For this review, use the dimensioned drawing (mm, ordinates from the lowest corner) and the shaded views. A direction names the side the tool comes from. Coordinates: 2 decimals unless noted, no trailing zeros. Loops run counter-clockwise (first coordinate to the right, second up) from the corner with the lowest first, then second, coordinate; pieces in that order, holes last.
1. Take a section at D-D, the plane x = 37. State the section outline as (y, z) points, then the cut area to 3 significant figures.
2. Take a section at B-B, the plane y = 2.3. State the section outline as (x, z) points.
3. Clearance check with flat-ended pins moving along their axes: P1, Ø1, axis at y = 2, z = 6, coming from the +X side; P2, Ø1, axis at y = 3.5, z = 13.5, coming from the +X side; P3, Ø3, axis at y = 0.5, z = 15.5, coming from the +X side. State where each tip first meets the part, or that it passes through.
4. Take a section at C-C, the plane z = 8.5. State the section outline as (x, y) points.
5. To check wall thickness, follow probe 1 along X at (y, z) = (1.05, 2); probe 2 along X at (y, z) = (3.15, 8.25); probe 3 along Z at (x, y) = (43, 1.9). State the ranges of each line that lie inside material, in increasing order.
6. Take a section at A-A, the plane z = 3.5. State the section outline as (x, y) points.
7. Machinability: for the marked faces 1, 2, 3, 4 and 5, which of the approach directions +Z, -Z, +X, -X, +Y, -Y give a long, thin tool a straight path to every point of the face, cutting with its end or side? Answer none if there is none.
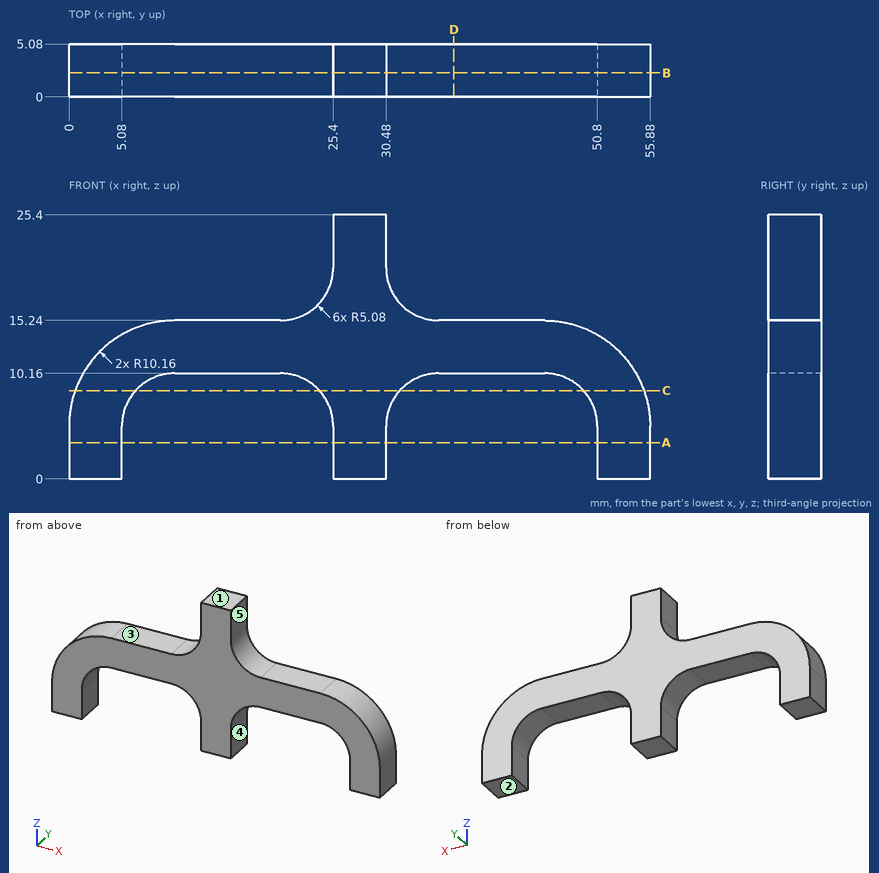
Results list:
1. outline: (0, 10.16) - (5.08, 10.16) - (5.08, 15.24) - (0, 15.24) - close
1. area: 25.8 mm2
2. outline: (0, 0) - (5.08, 0) - (5.08, 5.08) arc R5.08 cw to (10.16, 10.16) - (20.32, 10.16) arc R5.08 cw to (25.4, 5.08) - (25.4, 0) - (30.48, 0) - (30.48, 5.08) arc R5.08 cw to (35.56, 10.16) - (45.72, 10.16) arc R5.08 cw to (50.8, 5.08) - (50.8, 0) - (55.88, 0) - (55.88, 5.08) arc R10.16 ccw to (45.72, 15.24) - (35.56, 15.24) arc R5.08 cw to (30.48, 20.32) - (30.48, 25.4) - (25.4, 25.4) - (25.4, 20.32) arc R5.08 cw to (20.32, 15.24) - (10.16, 15.24) arc R10.16 ccw to (0, 5.08) - close
3. P1: stops at x = 55.87
3. P2: stops at x = 52.08
3. P3: stops at x = 50.58
4. outline: (0.59, 0) - (6.4, 0) - (6.4, 5.08) - (0.59, 5.08) - close; (24.08, 0) - (31.8, 0) - (31.8, 5.08) - (24.08, 5.08) - close; (49.48, 0) - (55.29, 0) - (55.29, 5.08) - (49.48, 5.08) - close
5. probe 1: x = 0 to 5.08, 25.4 to 30.48, 50.8 to 55.88
5. probe 2: x = 0.51 to 6.19, 24.29 to 31.59, 49.69 to 55.37
5. probe 3: z = 10.16 to 15.24
6. outline: (0, 0) - (5.08, 0) - (5.08, 5.08) - (0, 5.08) - close; (25.4, 0) - (30.48, 0) - (30.48, 5.08) - (25.4, 5.08) - close; (50.8, 0) - (55.88, 0) - (55.88, 5.08) - (50.8, 5.08) - close
7. face 1: +Z, +X, -X, +Y, -Y
7. face 2: -Z, +X, -X, +Y, -Y
7. face 3: +Z, -X, +Y, -Y
7. face 4: -Z, +Y, -Y
7. face 5: +Z, +X, +Y, -Y
